```python
from build123d import *

# Parameters (mm, degrees)
F1_DEPTH = 30
F2_R     = 7.5
F3_DEPTH = 22.9


with BuildPart() as f1:
    # F0 (on Front) → F1 (new body)
    with BuildSketch(Plane.XZ):
        with BuildLine():
            ThreePointArc((78.940095, 350), (98.415214, 340.67545), (103.362595, 319.657578))
            Line((103.362595, 319.657578), (40, 30))
            Line((40, 30), (40, 0))
            Line((40, 0), (40, -10))
            Line((40, -10), (50, -10))
            Line((50, -10), (50, 15))
            Line((50, 15), (60, 15))
            Line((60, 15), (60, -10))
            Line((60, -10), (70, -10))
            Line((70, -10), (70, 0))
            Line((70, 0), (70, 30))
            Line((70, 30), (170, 350))
            Line((170, 350), (170, 380))
            Line((170, 380), (0, 380))
            Line((0, 380), (0, 350))
            Line((0, 350), (78.940095, 350))
        make_face()
    extrude(amount=F1_DEPTH)

    # F2 (on face) → F3 (join)
    with BuildSketch(Plane.YZ.offset(70)):
        with Locations((-15, 0)):
            Circle(F2_R)
    extrude(amount=-F3_DEPTH)


solid = f1.part
```
Read the model definition and answer for the solid it produces. Units are mm, in the model's axes. A direction names the side the tool comes from. Give positions to 0.01 mm unless a question says otherwise; leave off trailing zeros. Order: outer loops, then holes, each group sorted by start corner. A loop starts at its lowest first (then second) coordinate and runs counter-clockwise, first axis right, second up.
(1) Find section B-B (z = 0). Give the vertices of the cut face in (x, y), plus the area to 3 significant figures.
(2) Find section D-D (z = 162.5). Give the vertices of the cut face in (x, y), plus the area to 3 significant figures.
(3) Straight lines are drawn through the part: L1, parallel to X at y = -17.5, z = 21; L2, parallel to X at y = -15.5, z = 176.5. For each, find the intervals that lie inside material, in ascending order.
(4) For a pull along Z with two mould halves and no side action, classify faces 4 (the flat face through (119.3, -14.79, 187.76)), 5 (the flat face through (60, -15, 8)), 6 (the flat face through (97, -30, 244)) as released by +Z, released by -Z, zero draft, split by the parting line, or undercut.
(5) Find section A-A (y = -15). Give the vertices of the cut face in (x, z), plus the area to 3 significant figures.
(6) Given pin 1 (3 mm diameter, centred on x = 54.5, y = -22.5, fed in from -Z); pin 2 (10 mm diameter, centred on x = 26.5, y = -11.5, fed in from -Z); pin 3 (7.5 mm diameter, centred on y = -8, z = 3.5, fed in from -X); pin 4 (2 mm diameter, centred on x = 57, z = 72, fed in from +Y), each flat-ended and moving along its own axis, determine where each tip first touches the part or whether it passes through.
(7) Find section C-C (x = 66.5). Give the vertices of the cut face in (y, z), plus the area to 3 significant figures.
(8) For faces 1 (the flat face through (50, -15, 8)), 2 (the flat face through (39, -15, 350)), 3 (the flat face through (55, -15, 15)), determine the directions among +Z, -Z, +X, -X, +Y, -Y from which every point of the face is accessible in a straight line to the end or side of a thin tool.
Result sheet:
1. outline: (40, -30) - (50, -30) - (50, -22.5) - (60, -22.5) - (60, -30) - (70, -30) - (70, 0) - (60, 0) - (60, -7.5) - (50, -7.5) - (50, 0) - (40, 0) - close
1. area: 750 mm2
2. outline: (68.98, -30) - (111.41, -30) - (111.41, 0) - (68.98, 0) - close
2. area: 1,270 mm2
3. L1: x = 40 to 70
3. L2: x = 72.05 to 115.78
4. face 4: released by -Z
4. face 5: undercut
4. face 6: zero draft
5. outline: (0, 350) - (78.94, 350) arc R25 cw to (103.36, 319.66) - (40, 30) - (40, -10) - (50, -10) - (50, -7.5) - (60, -7.5) - (60, -10) - (70, -10) - (70, 30) - (170, 350) - (170, 380) - (0, 380) - close; hole (50, 7.5) - (60, 7.5) - (60, 15) - (50, 15) - close
5. area: 20,800 mm2
6. pin 1: stops at z = -4.5
6. pin 2: stops at z = 350
6. pin 3: stops at x = 40
6. pin 4: stops at y = 0
7. outline: (-30, -10) - (0, -10) - (0, 151.14) - (-30, 151.14) - close; (-30, 350) - (0, 350) - (0, 380) - (-30, 380) - close
7. area: 5,730 mm2
8. face 1: none
8. face 2: -X, +Y, -Y
8. face 3: +Y, -Y
